Source: CAD feature listing. Evaluate the final solid. Frame: model axes, mm. A direction names the side the tool comes from. Round coordinates to 2 decimals unless told otherwise and drop trailing zeros. Loops run counter-clockwise (first coordinate to the right, second up) from the corner with the lowest first, then second, coordinate; pieces in that order, holes last. Notation, with made-up numbers: M -23,87 L -11,87 A18 cw -11,106 Z; hole C -34,76.5 d2. An arc over 180 degrees is marked long. One line per item, written item: value.
from build123d import *

# Parameters (mm, degrees)
SKETCH1_R               = 1.25
BOSS_EXTRUDE1_DEPTH     = 7
CUT_EXTRUDE1_DEPTH      = 63.812268863
CUT_EXTRUDE1_DEPTH_BACK = 63.812268863
SKETCH2_W               = 32.592394384
SKETCH2_H               = 3.5
FILLET1_R               = 5


with BuildPart() as part:
    # Sketch1 → Boss-Extrude1 (new body)
    with BuildSketch(Plane.XY):
        with BuildLine():
            Line((61.721813599, -1.473254022), (1.264188363, -5.267583503))
            Line((1.264188363, -5.267583503), (-8.846841125, -6.87670348))
            ThreePointArc((-8.846841125, -6.87670348), (-12.689755312, -4.606488283), (-11.177624454, -0.407044658))
            Line((-11.177624454, -0.407044658), (-1.302853294, 5.428691416))
            Line((-1.302853294, 5.428691416), (62.498270735, 1.424523457))
            Line((62.498270735, 1.424523457), (61.721813599, -1.473254022))
        make_face()
        Circle(SKETCH1_R, mode=Mode.SUBTRACT)
        with Locations((-9.396926208, -3.420201433)):
            Circle(SKETCH1_R, mode=Mode.SUBTRACT)
    extrude(amount=BOSS_EXTRUDE1_DEPTH)

    # Sketch2 → Cut-Extrude1 (cut, two sides: drawn at the far end of the back side and taken through both)
    with BuildSketch(Plane(origin=(0.427525179, -1.174615776, 0), x_dir=(0.9396926207859082, 0.3420201433256693, 0), z_dir=(-0.3420201433256693, 0.9396926207859082, 0)).offset(-CUT_EXTRUDE1_DEPTH_BACK)):
        with Locations((-12.046197192, -3.5)):
            Rectangle(SKETCH2_W, SKETCH2_H)
    extrude(amount=CUT_EXTRUDE1_DEPTH + CUT_EXTRUDE1_DEPTH_BACK, mode=Mode.SUBTRACT)

    # Fillet1
    # the kernel refuses this fillet: 5 mm, written as the material it adds along each edge
    with BuildSketch(Plane(origin=(1.264188363, -5.267583503, 5.25), x_dir=(0.9980363808193768, 0.06263691053172936, 0), z_dir=(0, 0, 1)), Plane(origin=(1.264188363, -5.267583503, 0), x_dir=(0.9980363808193768, 0.06263691053172936, 0), z_dir=(0, 0, 1))) as fillet1_piece_1:
        with BuildLine():
            CenterArc((FILLET1_R * 0.0476077036938, -FILLET1_R), FILLET1_R, 90, 5.45132501)
            Line((-FILLET1_R * 0.0473923866113, -FILLET1_R * 0.00452273615014), (0, 0))
            Line((0, 0), (FILLET1_R * 0.0476077036938, 0))
        make_face()
    extrude(amount=1.75)
    # the kernel refuses this fillet: 5 mm, written as the material it takes off along each edge
    with BuildSketch(Plane(origin=(-1.302853294, 5.428691416, 1.407700386), x_dir=(0.9980363808193763, -0.06263691053173732, 0), z_dir=(0, 0, 1))) as fillet1_2_piece_1:
        with BuildLine():
            CenterArc((FILLET1_R * 0.3073839691, -FILLET1_R), FILLET1_R, 90, 34.173177968)
            Line((-FILLET1_R * 0.254312163661, -FILLET1_R * 0.172656386716), (0, 0))
            Line((0, 0), (FILLET1_R * 0.3073839691, 0))
        make_face()
    extrude(amount=9.434599227, mode=Mode.SUBTRACT)
    with BuildSketch(Plane(origin=(-1.302853294, 5.428691416, -3.842299614), x_dir=(-0.8609019359097801, -0.5087709275762453, 0), z_dir=(0, 0, 1))) as fillet1_2_piece_2:
        with BuildLine():
            CenterArc((FILLET1_R * 0.3073839691, FILLET1_R), FILLET1_R, 235.826822032, 34.173177968)
            Line((-FILLET1_R * 0.254312163661, FILLET1_R * 0.172656386716), (0, 0))
            Line((0, 0), (FILLET1_R * 0.3073839691, 0))
        make_face()
    extrude(amount=9.434599227, mode=Mode.SUBTRACT)


solid = part.part
1. Pin query (flat end, axial travel): pin 1 (4 mm diameter, centred on x = 7.5, z = 2, fed in from +Y); pin 2 (2 mm diameter, centred on y = -0.5, z = 5, fed in from +X). Return the tip coordinate at first contact, or that it passes through.
Report:
pin 1: stops at y = 5
pin 2: stops at x = 62.25
2. Section query B-B (z = 3.25). Return the cut outline in (x, y), and give its area (3 significant figures).
Report:
outline: M 2.64,5.18 L 6.32,-4.95 L 61.72,-1.47 L 62.5,1.42 Z
area: 375 mm2
3. Ray query, line 1 (Y direction, x = 11, z = 1.25); line 2 (Y direction, x = 0, z = 0.85); line 3 (X direction, y = 0, z = 6.25). Return the intervals inside material, ascending. Write a range as [from, to].
Report:
line 1: y = [-4.66, 4.66]
line 2: y = [-5.47, -1.25], [1.25, 5.34]
line 3: x = [-10.49, -1.25], [1.25, 62.12]
4. Reachability of faces 1 (the face through (-3, -1, 5.25)), 2 (the face through (62.115, -0.004, 3.451)) from +Z, -Z, +X, -X, +Y, -Y: full face, straight path, thin tool, end or side. Return the list, or none.
Report:
face 1: -X, -Y
face 2: +Z, -Z, +X, -Y
5. Pull-direction query (Z, two-part tool) for faces 3 (the face through (4.51, 0.04, 3.52)), 4 (the face through (17, -1, 0)), 5 (the face through (-6.962, 2.084, 6.113)); classes: released by +Z, released by -Z, zero draft, split by the parting line, or undercut.
Report:
face 3: undercut
face 4: released by -Z
face 5: zero draft
6. Section query A-A (y = 3.75). Return the cut outline in (x, z), and give its area (3 significant figures).
Report:
outline: M -4.14,0 L 25.44,0 L 25.44,7 L -4.14,7 L -4.14,5.25 L 3.16,5.25 L 3.16,1.75 L -4.14,1.75 Z
area: 182 mm2
7. Section query C-C (x = 22). Return the cut outline in (y, z), and give its area (3 significant figures).
Report:
outline: M -3.97,0 L 3.97,0 L 3.97,7 L -3.97,7 Z
area: 55.5 mm2
